```python
from build123d import *

# Parameters (mm, degrees)
SKETCH1_R           = 2.5
BOSS_EXTRUDE1_DEPTH = 2.7


with BuildPart() as part:
    # Sketch1 → Boss-Extrude1 (new body)
    with BuildSketch(Plane.XY.offset(2.7)):
        Polygon((-2.309401077, 4), (-4.618802154, 0), (-2.309401077, -4), (2.309401077, -4), (4.618802154, 0), (2.309401077, 4), align=None)
        with Locations(Location((0, 0, 0), (0, 0, 180))):
            Circle(SKETCH1_R, mode=Mode.SUBTRACT)
    extrude(amount=-BOSS_EXTRUDE1_DEPTH)


solid = part.part
```
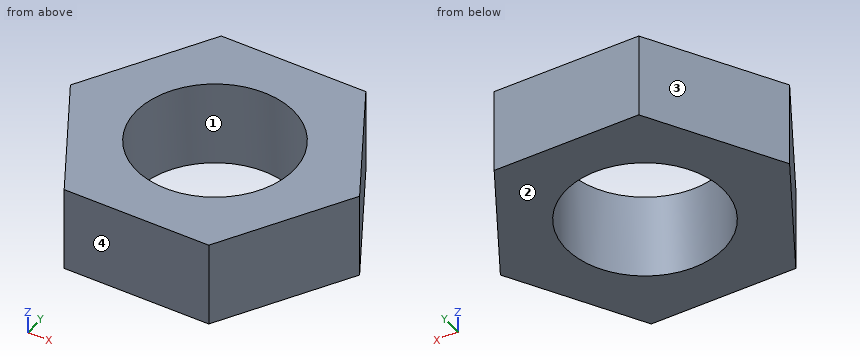
Geometry: final body of the model. Coordinates: model frame, mm. Face numbers are marked on the shaded views. Coordinates: 2 decimals unless noted, no trailing zeros. Order: outer loops, then holes, each group sorted by start corner. A loop starts at its lowest first (then second) coordinate and runs counter-clockwise, first axis right, second up.
Item 1: Contact query for flat-ended pins moving along their axis: P1, Ø1, axis at x = 1, y = 2, coming from the +Z side; P2, Ø1, axis at y = -1.5, z = 1.5, coming from the +X side. Output: stop coordinate, or through.
Answer:
P1: stops at z = 2.7
P2: stops at x = 4.04
Item 2: Section query A-A (x = 0). Output: boundary loops of the cut face in (y, z), then the cut area to 3 significant figures.
Answer:
outline: (-4, 0) - (-2.5, 0) - (-2.5, 2.7) - (-4, 2.7) - close; (2.5, 0) - (4, 0) - (4, 2.7) - (2.5, 2.7) - close
area: 8.10 mm2
Item 3: Section query C-C (y = 1.25). Output: boundary loops of the cut face in (x, z), then the cut area to 3 significant figures.
Answer:
outline: (-3.9, 0) - (-2.17, 0) - (-2.17, 2.7) - (-3.9, 2.7) - close; (2.17, 0) - (3.9, 0) - (3.9, 2.7) - (2.17, 2.7) - close
area: 9.35 mm2
Item 4: Section query D-D (x = 3.5). Output: boundary loops of the cut face in (y, z), then the cut area to 3 significant figures.
Answer:
outline: (-1.94, 0) - (1.94, 0) - (1.94, 2.7) - (-1.94, 2.7) - close
area: 10.5 mm2
Item 5: Section query B-B (z = 0.6). Output: boundary loops of the cut face in (x, y), then the cut area to 3 significant figures.
Answer:
outline: (-4.62, 0) - (-2.31, -4) - (2.31, -4) - (4.62, 0) - (2.31, 4) - (-2.31, 4) - close; hole circle Ø5 at (0, 0)
area: 35.8 mm2
Item 6: Material intervals for line 1 along Y through (x, z) = (0, 1.2); line 2 along Y through (x, z) = (-0.75, 1.8); line 3 along X through (y, z) = (2, 1.85), sorted ascending.
Answer:
line 1: y = -4 to -2.5, 2.5 to 4
line 2: y = -4 to -2.38, 2.38 to 4
line 3: x = -3.46 to -1.5, 1.5 to 3.46
Item 7: Draft query along Y for the marked faces 1, 2, 3 and 4. Return one class per face: released by +Y, released by -Y, zero draft, split by the parting line, or undercut.
Answer:
face 1: undercut
face 2: zero draft
face 3: released by +Y
face 4: released by -Y
